Here's how the part is built. I have some questions about the finished solid (model axes, mm). A direction names the side the tool comes from. Give positions to 0.01 mm unless a question says otherwise; leave off trailing zeros. Write each loop counter-clockwise with the first axis right and the second up, starting at its lowest first coordinate (ties: lowest second). Pieces come first, ordered by that corner, then holes. Notation, with made-up numbers: (42, -26.75) -> (85, -26.75) arc R14 ccw to (85, -9.75) -> close; hole circle Ø1 at (56.5, 1.25). An arc over 180 degrees is marked (long way). Use CSV: the item, a comma, the result in double quotes. Start each with the question number.
(1) Which directions (+Z, -Z, +X, -X, +Y, -Y) give clear straight access to the entire face, cutting with the end or side of a thin tool? Please do faces 1 (the cylindrical face through (366.58, 286.53, -14.26)), 2 (the flat face through (191.122, 154.035, -82.893)).
(2) Suppose I cut it at A-A on z = -87.5. List the corners of the cut face in (x, y) for me.
(3) Suppose I cut it at D-D on x = -263.5. List the corners of the cut face in (y, z) for me, plus the area to 3 significant figures.
(4) If we mould it in two halves opening along X, with no side actions, what happens to faces 3 (the flat face through (187.35, 144.8, -82.89)), 4 (the flat face through (-185.845, 149.956, -82.893)), 5 (the flat face through (-192.67, 148.91, -82.89))? For each: pulls with the +X half, pulls with the -X half, needs draft (parallel to the pull), parting line crosses it, or undercut.
(5) Suppose I cut it at C-C on z = -119.5. List the corners of the cut face in (x, y) for me, plus the area to 3 significant figures.
(6) Suppose I cut it at B-B on y = 168. List the corners of the cut face in (x, z) for me, plus the area to 3 significant figures.
(7) I need wall thicknesses on L1, parallel to X at y = 196, z = -61.5; L2, parallel to X at y = 152.5, z = -117.5; L3, parallel to Y at x = -185, z = -30. Which ranges of each line are inside material? Lowest first, please. Write a range as [from, to].
(8) For pin 1 Ø1.3 at (x, y) = (0.5, 1.5) entering from -Z; pin 2 Ø1.5 at (x, z) = (-238.5, -87.5) entering from +Y; pin 3 Ø1.5 at (x, z) = (178.5, -104.5) entering from +Y; pin 4 Ø1 at (x, z) = (-133.5, -128) entering from -Y, each with a flat end and sliding along its axis, tell me the tip position at first contact or that it passes through.
from build123d import *

# Parameters (mm, degrees)
BOSS_EXTRUDE1_DEPTH     = 240.2
CUT_EXTRUDE3_DEPTH      = 540.188032545
CUT_EXTRUDE3_DEPTH_BACK = 540.188032545
SKETCH2_W               = 760.049325768
SKETCH2_H               = 72.06
SKETCH3_W               = 12.4
SKETCH3_H               = 22.6
CUT_EXTRUDE4_DEPTH      = 512.167734023
FILLET1_R               = 50
SKETCH5_W               = 3
SKETCH5_H               = 33.628
CUT_EXTRUDE6_DEPTH      = 3


with BuildPart() as part:
    # Sketch1 → Boss-Extrude1 (new body)
    with BuildSketch(Plane.XY):
        Polygon((0, 0), (380.024662884, 293.716437401), (376.967027683, 297.672555066), (0, 6.319326703), (-376.967027683, 297.672555066), (-380.024662884, 293.716437401), align=None)
    extrude(amount=-BOSS_EXTRUDE1_DEPTH)

    # Sketch2 → Cut-Extrude3 (cut, two sides: drawn at the far end of the back side and taken through both)
    with BuildSketch(Plane(origin=(0, 0, 0), x_dir=(1, 0, 0), z_dir=(0, 1, 0)).offset(-CUT_EXTRUDE3_DEPTH_BACK)):
        with Locations((0, 204.17)):
            Rectangle(SKETCH2_W, SKETCH2_H)
    extrude(amount=CUT_EXTRUDE3_DEPTH + CUT_EXTRUDE3_DEPTH_BACK, mode=Mode.SUBTRACT)

    # Sketch3 → Cut-Extrude4 (cut, symmetric)
    with BuildSketch(Plane(origin=(3.057635201, 3.956117665, 0), x_dir=(0.7912235329674936, -0.6115270401858268, 0), z_dir=(0.6115270401858268, 0.7912235329674936, 0))):
        with Locations((-242.082219577, 143.14)):
            Rectangle(SKETCH3_W, SKETCH3_H)
    cut_extrude4 = extrude(amount=CUT_EXTRUDE4_DEPTH, both=True, mode=Mode.SUBTRACT)

    # Mirror1: Cut-Extrude4 across plane
    add(cut_extrude4.mirror(Plane(origin=(0, 0, 0), x_dir=(0, 0, 1), z_dir=(1, 0, 0))), mode=Mode.SUBTRACT)

    # Fillet1
    fillet1_edges = [part.edges().sort_by_distance(p)[0] for p in [
        (-378.495845284, 295.694496234, 0),
        (378.495845284, 295.694496234, 0),
    ]]
    fillet(fillet1_edges, radius=FILLET1_R)

    # Sketch5 → Cut-Extrude6 (cut)
    with BuildSketch(Plane(origin=(0, 0, 0), x_dir=(0.7912235329674936, -0.6115270401858267, 0), z_dir=(-0.6115270401858267, -0.7912235329674936, 0))):
        with Locations((-1.5, -16.814)):
            Rectangle(SKETCH5_W, SKETCH5_H)
        with Locations((-1.5, -84.07)):
            Rectangle(SKETCH5_W, SKETCH5_H)
        with Locations((-1.5, -151.326)):
            Rectangle(SKETCH5_W, SKETCH5_H)
    extrude(amount=-CUT_EXTRUDE6_DEPTH, mode=Mode.SUBTRACT)


solid = part.part
Geometry says:
1,face 1,"+Z, +X, +Y"
1,face 2,"+Z, -Z, +Y"
2,outline,"(-380.02, 293.72) -> (-2.37, 1.83) -> (-0.54, 4.21) -> (1.83, 2.37) -> (0, 0) -> (380.02, 293.72) -> (376.97, 297.67) -> (0, 6.32) -> (-376.97, 297.67) -> close"
3,outline,"(203.66, -168.14) -> (209.98, -168.14) -> (209.98, 0) -> (203.66, 0) -> close"
3,area,"1,060 mm²"
4,face 3,"pulls with the +X half"
4,face 4,"undercut"
4,face 5,"pulls with the -X half"
5,outline,"(-380.02, 293.72) -> (0, 0) -> (380.02, 293.72) -> (376.97, 297.67) -> (0, 6.32) -> (-376.97, 297.67) -> close"
5,area,"4,780 mm²"
6,outline,"(-217.37, -168.14) -> (-209.19, -168.14) -> (-209.19, 0) -> (-217.37, 0) -> close; (209.19, -168.14) -> (217.37, -168.14) -> (217.37, 0) -> (209.19, 0) -> close"
6,area,"2,750 mm²"
7,L1,"[-253.59, -245.42], [245.42, 253.59]"
7,L2,"[-197.31, -189.14], [189.14, 197.31]"
7,L3,"[142.98, 149.3]"
8,pin 1,"z = -168.14"
8,pin 2,"y = 191.23"
8,pin 3,"y = 144.86"
8,pin 4,"y = 102.79"
